```python
from build123d import *

# Parameters (mm, degrees)
SKETCH1_W           = 50
SKETCH1_H           = 36
BOSS_EXTRUDE1_DEPTH = 24
SHELL1_T            = 1.5
SKETCH2_W           = 4
SKETCH2_H           = 36
BOSS_EXTRUDE2_DEPTH = 18
SKETCH6_W           = 14
SKETCH6_H           = 14
CUT_EXTRUDE2_DEPTH  = 10
FILLET1_R           = 3
SKETCH4_R           = 3
BOSS_EXTRUDE3_DEPTH = 18
SKETCH7_R           = 1.6
CUT_EXTRUDE3_DEPTH  = 12
SKETCH8_W           = 33
SKETCH8_H           = 8
CUT_EXTRUDE4_DEPTH  = 5
FILLET3_R           = 7


with BuildPart() as part:
    # Sketch1 → Boss-Extrude1 (new body)
    with BuildSketch(Plane(origin=(0, 0, 0), x_dir=(1, 0, 0), z_dir=(0, 1, 0))):
        with Locations((25, -18)):
            Rectangle(SKETCH1_W, SKETCH1_H)
    extrude(amount=BOSS_EXTRUDE1_DEPTH)

    # Shell1
    shell1_openings = [part.faces().sort_by_distance(p)[0] for p in [
        (25, 24, 18),
    ]]
    offset(amount=SHELL1_T, openings=shell1_openings, kind=Kind.INTERSECTION)

    # Sketch2 → Boss-Extrude2 (add)
    with BuildSketch(Plane(origin=(0, 0, 0), x_dir=(1, 0, 0), z_dir=(0, 1, 0))):
        with Locations((7, -18)):
            Rectangle(SKETCH2_W, SKETCH2_H)
        with Locations((43, -18)):
            Rectangle(SKETCH2_W, SKETCH2_H)
    extrude(amount=BOSS_EXTRUDE2_DEPTH)

    # Sketch6 → Cut-Extrude2 (cut)
    with BuildSketch(Plane.XY.offset(37.5)):
        with Locations((25, 21.134691447)):
            Rectangle(SKETCH6_W, SKETCH6_H)
    extrude(amount=-CUT_EXTRUDE2_DEPTH, mode=Mode.SUBTRACT)

    # Fillet1
    fillet1_edges = [part.edges().sort_by_distance(p)[0] for p in [
        (0, 12, 0),
        (0, 12, 36),
        (50, 12, 36),
        (50, 12, 0),
        (32, 24, 36.75),
        (18, 24, 36.75),
        (18, 14.134691447, 36.75),
        (32, 14.134691447, 36.75),
    ]]
    fillet(fillet1_edges, radius=FILLET1_R)

    # Sketch4 → Boss-Extrude3 (add)
    with BuildSketch(Plane(origin=(0, 18, 0), x_dir=(1, 0, 0), z_dir=(0, 1, 0))):
        with Locations((7, -16)):
            Circle(SKETCH4_R)
        with Locations((43, -16)):
            Circle(SKETCH4_R)
    extrude(amount=-BOSS_EXTRUDE3_DEPTH)

    # Sketch7 → Cut-Extrude3 (cut)
    with BuildSketch(Plane(origin=(0, 18, 0), x_dir=(1, 0, 0), z_dir=(0, 1, 0))):
        with Locations(Location((7, -16, 0), (0, 0, 270))):
            Circle(SKETCH7_R)
        with Locations(Location((43, -16, 0), (0, 0, 90))):
            Circle(SKETCH7_R)
    extrude(amount=-CUT_EXTRUDE3_DEPTH, mode=Mode.SUBTRACT)

    # Sketch8 → Cut-Extrude4 (cut)
    with BuildSketch(Plane(origin=(0, 0, -1.5), x_dir=(-1, 0, 0), z_dir=(0, 0, -1))):
        with Locations((-25, 22)):
            Rectangle(SKETCH8_W, SKETCH8_H)
    extrude(amount=-CUT_EXTRUDE4_DEPTH, mode=Mode.SUBTRACT)

    # Fillet3
    # the kernel refuses this fillet: 7 mm, written as the material it takes off along each edge
    with BuildSketch(Plane(origin=(41.5, 24, -18.820508076), x_dir=(0, -1, 0), z_dir=(0, 0, 1))) as fillet3_piece_1:
        with BuildLine():
            CenterArc((7, 6.92820323), FILLET3_R, 180, 81.786789298)
            Line((0, 6.92820323), (-0.14, 6.92820323))
            Line((-0.14, 6.92820323), (-0.14, 0))
            Line((-0.14, 0), (0, -0.14))
            ThreePointArc((0, -0.14), (3, -0.14), (5.98, -0.138564065))
            Line((5.98, -0.138564065), (6, 0))
        make_face()
    extrude(amount=36.141016151, mode=Mode.SUBTRACT)
    with BuildSketch(Plane(origin=(8.5, 24, 17.320508076), x_dir=(-1, 0, 0), z_dir=(0, 0, -1))) as fillet3_piece_2:
        with BuildLine():
            CenterArc((6.92820323, -7), FILLET3_R, 90, 81.786789298)
            Line((0, -6), (-0.138564065, -5.98))
            ThreePointArc((-0.138564065, -5.98), (-0.14, -3), (-0.14, 0))
            Line((-0.14, 0), (0, 0.14))
            Line((0, 0.14), (6.92820323, 0.14))
            Line((6.92820323, 0.14), (6.92820323, 0))
        make_face()
    extrude(amount=36.141016151, mode=Mode.SUBTRACT)


solid = part.part
```
The model under review builds one solid part; all positions refer to its coordinate system, in mm. A direction names the side the tool comes from. Coordinates: 2 decimals unless noted, no trailing zeros. Write each loop counter-clockwise with the first axis right and the second up, starting at its lowest first coordinate (ties: lowest second). Pieces come first, ordered by that corner, then holes.
1) We need section B-B on z = 13. State the section outline as (x, y) points, then the cut area to 4 significant figures.
2) The part is to be moulded in two halves that separate along Z. For faces 1 (the face through (50, 12, 18)), 2 (the face through (-1.5, 11, 18)), 3 (the face through (25, 11, 37.5)), 4 (the face through (5, 9, 27)), say which applies: pulls with the +Z half, pulls with the -Z half, needs draft (parallel to the pull), parting line crosses it, or undercut.
3) Machinability: for faces 5 (the face through (25, 14.135, 37)), 6 (the face through (51, 24, 22)), 7 (the face through (25, 12, 36)), which of the approach directions +Z, -Z, +X, -X, +Y, -Y give a long, thin tool a straight path to every point of the face, cutting with its end or side? Answer none if there is none.
4) We need section C-C on x = 11.5. State the section outline as (y, z) points.
5) To check wall thickness, follow probe 1 along X at (y, z) = (16.75, 31); probe 2 along X at (y, z) = (11.75, 16); probe 3 along Z at (x, y) = (43, 10). State the ranges of each line that lie inside material, in increasing order.
6) We need section D-D on z = 1. State the section outline as (x, y) points.
7) We need section A-A on y = 16.25. Count the separate pieces of the cut face and the enclosed holes in it, then the cut area to 3 significant figures.
8) Clearance check with flat-ended pins moving along their axes: pin 1 Ø3.5 at (x, z) = (6, 16.5) entering from +Y; pin 2 Ø0.8 at (x, z) = (23, 37) entering from +Y; pin 3 Ø2 at (x, y) = (23, 17.5) entering from +Z. State where each tip first meets the part, or that it passes through.
Answer list:
1. outline: (-1.5, -1.5) - (51.5, -1.5) - (51.5, 24) - (50, 24) - (50, 0) - (45, 0) - (45, 18) - (41, 18) - (41, 0) - (9, 0) - (9, 18) - (5, 18) - (5, 0) - (0, 0) - (0, 24) - (-1.5, 24) - close
1. area: 295.5 mm2
2. face 1: undercut
2. face 2: needs draft
2. face 3: pulls with the +Z half
2. face 4: undercut
3. face 5: +Z, +Y
3. face 6: +Z, -Z, +X, -X, +Y
3. face 7: +Y
4. outline: (-1.5, -1.5) - (18, -1.5) - (18, 0) - (0, 0) - (0, 36) - (24, 36) - (24, 37.5) - (-1.5, 37.5) - close
5. probe 1: x = -1.5 to 0, 5 to 9, 41 to 45, 50 to 51.5
5. probe 2: x = -1.5 to 0, 4 to 5.4, 8.6 to 10, 40 to 41.4, 44.6 to 46, 50 to 51.5
5. probe 3: z = -1.5 to 14.4, 17.6 to 37.5
6. outline: (-1.5, -1.5) - (51.5, -1.5) - (51.5, 24) - (49.24, 24) - (49.24, 0) - (45, 0) - (45, 18) - (41, 18) - (41, 0) - (9, 0) - (9, 18) - (5, 18) - (5, 0) - (0.76, 0) - (0.76, 24) - (-1.5, 24) - close
7. separate pieces: 1
7. enclosed holes: 4
7. area: 538 mm2
8. pin 1: stops at y = 18
8. pin 2: stops at y = 14.13
8. pin 3: stops at z = 0
